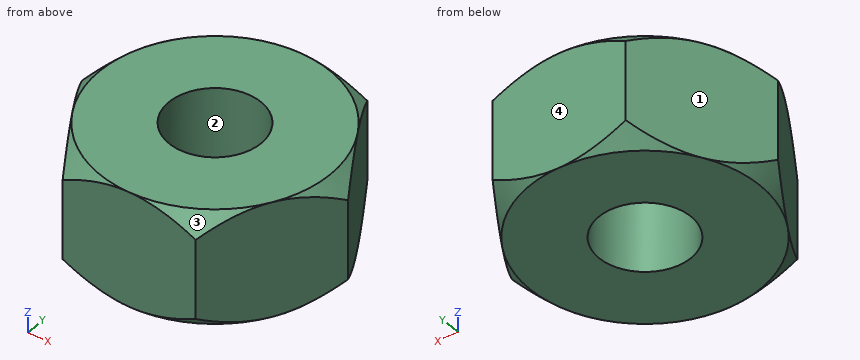
from build123d import *

# Parameters (mm, degrees)
IZIM1_R                     = 2
Y_KSEKLIK_EKSTR_ZYON1_DEPTH = 5
IZIM2_OUTSIDE_W             = 18.762
IZIM2_OUTSIDE_H             = 17.214
IZIM2_OUTSIDE_R             = 5
KES_EKSTR_ZYON1_DEPTH       = 1
KES_EKSTR_ZYON1_DRAFT       = -45
IZIM3_OUTSIDE_W             = 18.762
IZIM3_OUTSIDE_H             = 17.214
IZIM3_OUTSIDE_R             = 5
KES_EKSTR_ZYON2_DEPTH       = 1
KES_EKSTR_ZYON2_DRAFT       = -45


with BuildPart() as part:
    # Çizim1 → Yükseklik-Ekstrüzyon1 (new body)
    with BuildSketch(Plane.XY):
        Polygon((5.773502692, 0), (2.886751346, 5), (-2.886751346, 5), (-5.773502692, 0), (-2.886751346, -5), (2.886751346, -5), align=None)
        Circle(IZIM1_R, mode=Mode.SUBTRACT)
    extrude(amount=Y_KSEKLIK_EKSTR_ZYON1_DEPTH)


with BuildPart() as kes_ekstr_zyon1_tool:
    # Çizim2 outside → Kes-Ekstrüzyon1 (with draft: the straight prism first)
    with BuildSketch(Plane.XY.offset(5)):
        Rectangle(IZIM2_OUTSIDE_W, IZIM2_OUTSIDE_H)
        Circle(IZIM2_OUTSIDE_R, mode=Mode.SUBTRACT)
    extrude(amount=-KES_EKSTR_ZYON1_DEPTH)
    # Kes-Ekstrüzyon1: the draft: its side faces are tilted about the plane it starts from
    kes_ekstr_zyon1_sides = [kes_ekstr_zyon1_tool.faces().sort_by_distance(p)[0] for p in [
        (0, -8.607, 4.5),
        (9.381, 0, 4.5),
        (0, 8.607, 4.5),
        (-9.381, 0, 4.5),
        (-5, 0, 4.5),
    ]]
    draft(kes_ekstr_zyon1_sides, Plane.XY.offset(5), KES_EKSTR_ZYON1_DRAFT)


with BuildPart() as part_1:
    add(part.part)

    # Kes-Ekstrüzyon1: cut by kes_ekstr_zyon1_tool
    add(kes_ekstr_zyon1_tool.part, mode=Mode.SUBTRACT)


with BuildPart() as kes_ekstr_zyon2_tool:
    # Çizim3 outside → Kes-Ekstrüzyon2 (with draft: the straight prism first)
    with BuildSketch(Plane(origin=(0, 0, 0), x_dir=(-1, 0, 0), z_dir=(0, 0, -1))):
        Rectangle(IZIM3_OUTSIDE_W, IZIM3_OUTSIDE_H)
        Circle(IZIM3_OUTSIDE_R, mode=Mode.SUBTRACT)
    extrude(amount=-KES_EKSTR_ZYON2_DEPTH)
    # Kes-Ekstrüzyon2: the draft: its side faces are tilted about the plane it starts from
    kes_ekstr_zyon2_sides = [kes_ekstr_zyon2_tool.faces().sort_by_distance(p)[0] for p in [
        (0, -8.607, 0.5),
        (-9.381, 0, 0.5),
        (0, 8.607, 0.5),
        (9.381, 0, 0.5),
        (5, 0, 0.5),
    ]]
    draft(kes_ekstr_zyon2_sides, Plane(origin=(0, 0, 0), x_dir=(-1, 0, 0), z_dir=(0, 0, -1)), KES_EKSTR_ZYON2_DRAFT)


with BuildPart() as part_2:
    add(part_1.part)

    # Kes-Ekstrüzyon2: cut by kes_ekstr_zyon2_tool
    add(kes_ekstr_zyon2_tool.part, mode=Mode.SUBTRACT)


solid = part_2.part
Can you work these out from the model? Positions are in its coordinate system, mm. Face numbers are marked on the shaded views. Coordinates: 2 decimals unless noted, no trailing zeros. Loops run counter-clockwise (first coordinate to the right, second up) from the corner with the lowest first, then second, coordinate; pieces in that order, holes last. Notation, with made-up numbers: (24, 4) - (41, 4) arc R22 cw to (41, 32) - close; hole circle Ø9 at (-6, -21.5). An arc over 180 degrees is marked (long way). Put each result on its own line as item: value. Start each with the question number.
Item 1: Suppose I cut it at A-A (z = 2.95). Please give me the cut outline in (x, y).
Item 2: For pin 1 (1 mm diameter, centred on y = 2.5, z = 4, fed in from -X); pin 2 (1 mm diameter, centred on x = 4.5, z = 1, fed in from +Y), each with a flat end and sliding along its axis, tell me the tip position at first contact or that it passes through.
Item 3: If I drill on line 1 along Y through (x, z) = (-0.75, 4.6); line 2 along X through (y, z) = (0.75, 4.4); line 3 along X through (y, z) = (-0.5, 2.05), over which ranges is the centre line in solid material (lowest first)?
Item 4: If we mould it in two halves opening along X, with no side actions, what happens to the marked faces 1, 2, 3 and 4? For each: +X half, -X half, draft (parallel to the pull), parting line (faces both ways), or undercut.
Item 5: Suppose I cut it at B-B (z = 4.4). Please give me the cut outline in (x, y).
Here are the results:
1. outline: (-5.77, 0) - (-2.89, -5) - (2.89, -5) - (5.77, 0) - (2.89, 5) - (-2.89, 5) - close; hole circle Ø4 at (0, 0)
2. pin 1: x = -4.62
2. pin 2: y = 3.07
3. line 1: -5 to -1.85, 1.85 to 5
3. line 2: -5.34 to -1.85, 1.85 to 5.34
3. line 3: -5.48 to -1.94, 1.94 to 5.48
4. face 1: -X half
4. face 2: undercut
4. face 3: +X half
4. face 4: draft
5. outline: (-5.59, -0.32) - (-3.07, -4.68) arc R5.6 ccw to (-2.52, -5) - (2.52, -5) arc R5.6 ccw to (3.07, -4.68) - (5.59, -0.32) arc R5.6 ccw to (5.59, 0.32) - (3.07, 4.68) arc R5.6 ccw to (2.52, 5) - (-2.52, 5) arc R5.6 ccw to (-3.07, 4.68) - (-5.59, 0.32) arc R5.6 ccw to start; hole circle Ø4 at (0, 0)
